Design review of the part built by this model. Coordinates are the model's own, in mm. A direction names the side the tool comes from. Coordinates: 2 decimals unless noted, no trailing zeros. Loops run counter-clockwise (first coordinate to the right, second up) from the corner with the lowest first, then second, coordinate; pieces in that order, holes last. Notation, with made-up numbers: (-10.75, 13.5) -> (-2.75, 13.5) arc R28 cw to (-2.75, 49.5) -> close; hole circle Ø10 at (38.5, -38.5). An arc over 180 degrees is marked (long way). Answer as a JSON object with one key per item and string values.
```python
from build123d import *

# Parameters (mm, degrees)
SKETCH_1_R          = 20
EXTRUDE_1_DEPTH     = 4
SKETCH_2_R          = 10
EXTRUDE_2_DEPTH     = 11.2
SKETCH_3_R          = 1.5
CUT_EXTRUDE_1_DEPTH = 31.421045347
SKETCH_4_R          = 8.5
EXTRUDE_3_DEPTH     = 25
SKETCH_5_R          = 5
CUT_EXTRUDE_2_DEPTH = 50.153229802
SKETCH_6_W          = 0.8
SKETCH_6_H          = 1
CHAMFER_1_SIZE      = 0.5


with BuildPart() as part:
    # 草图1 → 凸台-拉伸1 (new body)
    with BuildSketch(Plane(origin=(0, 0, 0), x_dir=(1, 0, 0), z_dir=(0, 1, 0))):
        with Locations(Location((0, 0, 0), (0, 0, 270))):
            Circle(SKETCH_1_R)
    extrude(amount=EXTRUDE_1_DEPTH)

    # 草图2 → 凸台-拉伸2 (add)
    with BuildSketch(Plane(origin=(0, 4, 0), x_dir=(1, 0, 0), z_dir=(0, 1, 0))):
        with Locations(Location((0, 0, 0), (0, 0, 270))):
            Circle(SKETCH_2_R)
    extrude(amount=EXTRUDE_2_DEPTH)

    # 草图3 → 切除-拉伸1 (cut, through all)
    with BuildSketch(Plane(origin=(0, 4, 0), x_dir=(1, 0, 0), z_dir=(0, 1, 0))):
        with Locations(Location((0, 17.5, 0), (0, 0, 270))):
            Circle(SKETCH_3_R)
        with Locations(Location((12.374368671, 12.374368671, 0), (0, 0, 270))):
            Circle(SKETCH_3_R)
        with Locations(Location((17.5, 0, 0), (0, 0, 270))):
            Circle(SKETCH_3_R)
        with Locations(Location((12.374368671, -12.374368671, 0), (0, 0, 270))):
            Circle(SKETCH_3_R)
        with Locations(Location((0, -17.5, 0), (0, 0, 270))):
            Circle(SKETCH_3_R)
        with Locations(Location((-12.374368671, -12.374368671, 0), (0, 0, 270))):
            Circle(SKETCH_3_R)
        with Locations(Location((-17.5, 0, 0), (0, 0, 270))):
            Circle(SKETCH_3_R)
        with Locations(Location((-12.374368671, 12.374368671, 0), (0, 0, 270))):
            Circle(SKETCH_3_R)
    extrude(amount=-CUT_EXTRUDE_1_DEPTH, mode=Mode.SUBTRACT)

    # 草图4 → 凸台-拉伸3 (add)
    with BuildSketch(Plane(origin=(0, 15.2, 0), x_dir=(1, 0, 0), z_dir=(0, 1, 0))):
        with Locations(Location((0, 0, 0), (0, 0, 270))):
            Circle(SKETCH_4_R)
    extrude(amount=EXTRUDE_3_DEPTH)

    # 草图5 → 切除-拉伸2 (cut, through all)
    with BuildSketch(Plane(origin=(0, 40.2, 0), x_dir=(1, 0, 0), z_dir=(0, 1, 0))):
        with Locations(Location((0, 0, 0), (0, 0, 270))):
            Circle(SKETCH_5_R)
    extrude(amount=-CUT_EXTRUDE_2_DEPTH, mode=Mode.SUBTRACT)

    # 草图6 → 切除-旋转1 (revolve, cut)
    with BuildSketch(Plane.XY, mode=Mode.PRIVATE) as cut_revolve_1_sk:
        with Locations((8.1, 37.7)):
            Rectangle(SKETCH_6_W, SKETCH_6_H)
    revolve(cut_revolve_1_sk.sketch.rotate(Axis((0, 40.2, 0), (0, -1, 0)), 90), axis=Axis((0, 40.2, 0), (0, -1, 0)), mode=Mode.SUBTRACT)

    # 倒角1
    chamfer_1_edges = [part.edges().sort_by_distance(p)[0] for p in [
        (0, 40.2, -8.5),
        (0, 15.2, -10),
    ]]
    chamfer(chamfer_1_edges, length=CHAMFER_1_SIZE)


solid = part.part
```
1) Clearance check with flat-ended pins moving along their axes: pin 1 Ø4 at (x, y) = (9, 23) entering from +Z; pin 2 Ø4 at (x, z) = (17.5, 0) entering from +Y; pin 3 Ø1 at (y, z) = (5, -8.5) entering from -X. State where each tip first meets the part, or that it passes through.
Completed:
{"pin 1": "z = 4.82", "pin 2": "y = 4", "pin 3": "x = -6"}
2) Add section D-D, the plane z = -12.5. Give the boundary of the cut face in (x, y), and give its area (3 significant figures).
Completed:
{"outline": "(-15.61, 0) -> (-13.87, 0) -> (-13.87, 4) -> (-15.61, 4) -> close; (-10.88, 0) -> (10.88, 0) -> (10.88, 4) -> (-10.88, 4) -> close; (13.87, 0) -> (15.61, 0) -> (15.61, 4) -> (13.87, 4) -> close", "area": "101 mm²"}
3) Add section C-C, the plane y = 8.5. Give the boundary of the cut face in (x, z).
Completed:
{"outline": "circle Ø20 at (0, 0); hole circle Ø10 at (0, 0)"}
4) For faces 1 (the flat face through (9, 4, -5)), 2 (the flat face through (-8, 38.2, 1)), 3 (the cylindrical face through (0, 2, 16)), list the 3-axis set-ups (+Z, -Z, +X, -X, +Y, -Y) from which the entire face can be reached by the end or side of a thin tool; tool diameter is ignored.
Completed:
{"face 1": "+Y", "face 2": "none", "face 3": "+Y, -Y"}
5) Add section A-A, the plane x = -17.5. Give the boundary of the cut face in (y, z).
Completed:
{"outline": "(0, -9.68) -> (4, -9.68) -> (4, -1.5) -> (0, -1.5) -> close; (0, 1.5) -> (4, 1.5) -> (4, 9.68) -> (0, 9.68) -> close"}
6) Wall thickness on probe 1 along X at (y, z) = (1.95, 0); probe 2 along Y at (x, z) = (-5.5, -5.5); probe 3 along X at (y, z) = (13.5, 0): over which ranges is each line inside the solid? List them lowest first.
Completed:
{"probe 1": "-20 to -19, -16 to -5, 5 to 16, 19 to 20", "probe 2": "0 to 37.2, 38.2 to 40.2", "probe 3": "-10 to -5, 5 to 10"}
7) The part is to be moulded in two halves that separate along Z. For faces 4 (the cylindrical face through (11.8, 2.03, 13.76)), 5 (the flat face through (-8, 37.2, 1)), 6 (the cylindrical face through (10.91, 2.03, -12.7)), 7 (the cylindrical face through (8.428, 38.94, -1.107)), say which applies: pulls with the +Z half, pulls with the -Z half, needs draft (parallel to the pull), parting line crosses it, or undercut.
Completed:
{"face 4": "undercut", "face 5": "needs draft", "face 6": "undercut", "face 7": "parting line crosses it"}
8) Add section B-B, the plane z = -17.5. Give the boundary of the cut face in (x, y), and give its area (3 significant figures).
Completed:
{"outline": "(-9.68, 0) -> (-1.5, 0) -> (-1.5, 4) -> (-9.68, 4) -> close; (1.5, 0) -> (9.68, 0) -> (9.68, 4) -> (1.5, 4) -> close", "area": "65.5 mm²"}
